Input: part model. Units: mm. Frame: model coordinates. Face numbers are marked on the shaded views. Give positions to 0.01 mm unless a question says otherwise; leave off trailing zeros. Loops run counter-clockwise (first coordinate to the right, second up) from the corner with the lowest first, then second, coordinate; pieces in that order, holes last. Notation, with made-up numbers: (19, 73) -> (65, 73) arc R27 cw to (65, 92) -> close; hole circle Ø5 at (-1.75, 65.25). An arc over 180 degrees is marked (long way). Use CSV: the item, a comma, the result in double quotes.
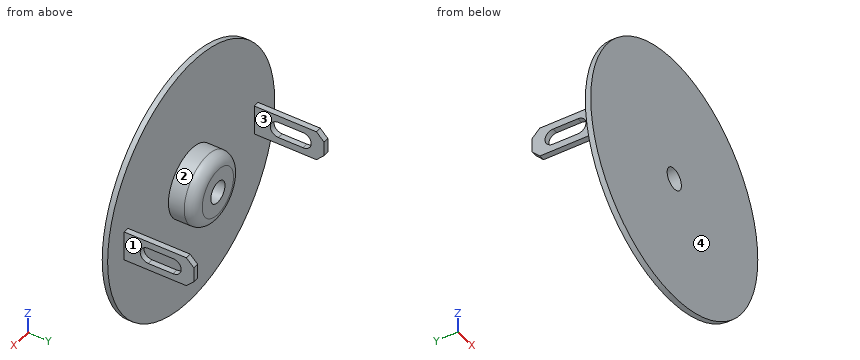
```python
from build123d import *

# Parameters (mm, degrees)
SKETCH_1_R                 = 11.75
SKETCH_1_R_2               = 1
EXTRUDE_1_DEPTH            = 0.5
SKETCH_2_W                 = 0.53
SKETCH_2_H                 = 2.78
EXTRUDE_2_DEPTH            = 6.42
CHAMFER_1_SIZE             = 0.7
CUT_EXTRUDE_1_DEPTH        = 0.53
SKETCH_4_W                 = 2.2
SKETCH_4_H                 = 2.46
FILLET_1_R                 = 1
CHAMFER_1_OF_MIRROR_1_SIZE = 0.7


with BuildPart() as part:
    # 草图1 → 凸台-拉伸1 (new body)
    with BuildSketch(Plane(origin=(0, 0, 0), x_dir=(1, 0, 0), z_dir=(0, 1, 0))):
        Circle(SKETCH_1_R)
        Circle(SKETCH_1_R_2, mode=Mode.SUBTRACT)
    extrude(amount=EXTRUDE_1_DEPTH)

    # 草图2 → 凸台-拉伸2 (add)
    with BuildSketch(Plane(origin=(0, 0.5, 0), x_dir=(1, 0, 0), z_dir=(0, 1, 0))):
        with Locations((-9.15, 0)):
            Rectangle(SKETCH_2_W, SKETCH_2_H)
    extrude_2 = extrude(amount=EXTRUDE_2_DEPTH)

    # 倒角1
    chamfer_1_edges = [part.edges().sort_by_distance(p)[0] for p in [
        (-9.15, 6.92, -1.39),
        (-9.15, 6.92, 1.39),
    ]]
    chamfer(chamfer_1_edges, length=CHAMFER_1_SIZE)

    # 草图3 → 切除-拉伸1 (cut)
    with BuildSketch(Plane.ZY.offset(9.415)):
        with BuildLine():
            Line((0.751927557, 4.991992343), (0.751927557, 2.722407652))
            ThreePointArc((0.751927557, 2.722407652), (0, 1.970480095), (-0.751927557, 2.722407652))
            Line((-0.751927557, 2.722407652), (-0.751927557, 4.991992343))
            ThreePointArc((-0.751927557, 4.991992343), (0, 5.7439199), (0.751927557, 4.991992343))
        make_face()
    cut_extrude_1 = extrude(amount=-CUT_EXTRUDE_1_DEPTH, mode=Mode.SUBTRACT)

    # 草图4 → 旋转1 (revolve)
    with BuildSketch(Plane.XY):
        with Locations((-2.1, 1.73)):
            Rectangle(SKETCH_4_W, SKETCH_4_H)
    revolve(axis=Axis((0, 3.495676189, 0), (0, -1, 0)))

    # 圆角1
    fillet_1_edges = [part.edges().sort_by_distance(p)[0] for p in [
        (3.2, 2.96, 0),
    ]]
    fillet(fillet_1_edges, radius=FILLET_1_R)

    # 镜向1: 凸台-拉伸2, 切除-拉伸1 across plane
    add(extrude_2.mirror(Plane(origin=(0, 0, 0), x_dir=(0, 0, 1), z_dir=(1, 0, 0))))
    add(cut_extrude_1.mirror(Plane(origin=(0, 0, 0), x_dir=(0, 0, 1), z_dir=(1, 0, 0))), mode=Mode.SUBTRACT)

    # 倒角1 of 镜向1
    chamfer_1_of_mirror_1_edges = [part.edges().sort_by_distance(p)[0] for p in [
        (9.15, 6.92, -1.39),
        (9.15, 6.92, 1.39),
    ]]
    chamfer(chamfer_1_of_mirror_1_edges, length=CHAMFER_1_OF_MIRROR_1_SIZE)


solid = part.part
```
1) Ray query, line 1 (X direction, y = 0.7, z = 0) (3 decimals); line 2 (Z direction, x = 0, y = 1); line 3 (Y direction, x = -1.5, z = -1.5). Return the intervals inside material, ascending.
From the geometry:
line 1,"x = -9.415 to -8.885, -3.2 to -1, 1 to 3.2, 8.885 to 9.415"
line 2,"z = -3.2 to -1, 1 to 3.2"
line 3,"y = 0 to 2.96"
2) Contact query for flat-ended pins moving along their axis: pin 1 (3 mm diameter, centred on x = -1, z = 6, fed in from -Y); pin 2 (3.5 mm diameter, centred on x = 0.5, z = 0.5, fed in from +Y); pin 3 (7 mm diameter, centred on x = 4.5, z = 4.5, fed in from +Y); pin 4 (2 mm diameter, centred on y = 4.5, z = -0.5, fed in from +X) (3 decimals). Output: stop coordinate, or through.
From the geometry:
pin 1,"stops at y = 0"
pin 2,"stops at y = 2.96"
pin 3,"stops at y = 2.71"
pin 4,"stops at x = 9.415"
3) Section query C-C (x = 0). Return loops of the section in (y, z).
From the geometry:
outline,"(0, -11.75) -> (0.5, -11.75) -> (0.5, -3.2) -> (1.96, -3.2) arc R1 ccw to (2.96, -2.2) -> (2.96, -1) -> (0, -1) -> close; (0, 1) -> (2.96, 1) -> (2.96, 2.2) arc R1 ccw to (1.96, 3.2) -> (0.5, 3.2) -> (0.5, 11.75) -> (0, 11.75) -> close"
4) Section query B-B (z = 0). Give the number of separate pieces and of enclosed holes in the cut face, then the cut area to 3 significant figures.
From the geometry:
separate pieces,"4"
enclosed holes,"0"
area,"24.0 mm^2"
5) Section query D-D (z = -8). Return loops of the section in (x, y).
From the geometry:
outline,"(-8.61, 0) -> (8.61, 0) -> (8.61, 0.5) -> (-8.61, 0.5) -> close"
6) Section query A-A (y = 4.5). Return loops of the section in (x, z) (3 decimals), then the cut area to 3 significant figures.
From the geometry:
outline,"(-9.415, -1.39) -> (-8.885, -1.39) -> (-8.885, -0.752) -> (-9.415, -0.752) -> close; (-9.415, 0.752) -> (-8.885, 0.752) -> (-8.885, 1.39) -> (-9.415, 1.39) -> close; (8.885, -1.39) -> (9.415, -1.39) -> (9.415, -0.752) -> (8.885, -0.752) -> close; (8.885, 0.752) -> (9.415, 0.752) -> (9.415, 1.39) -> (8.885, 1.39) -> close"
area,"1.35 mm^2"
7) Mould query, pull axis X, two halves, no side actions, for the marked faces 1, 2, 3 and 4. Classes: pulls with the +X half, pulls with the -X half, needs draft (parallel to the pull), parting line crosses it, or undercut.
From the geometry:
face 1,"pulls with the +X half"
face 2,"undercut"
face 3,"undercut"
face 4,"needs draft"
